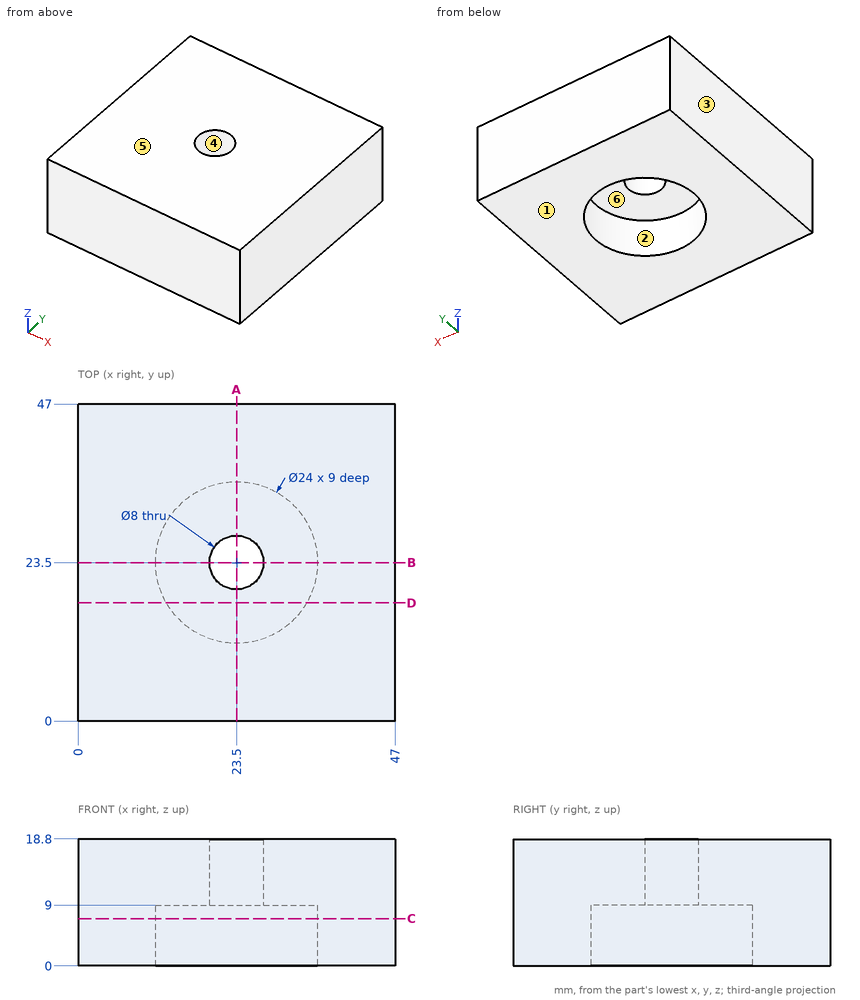
Design review of the part shown in the three views and the two pictorial views. Dimensions are in mm from the part's minimum x, y and z. A direction names the side the tool comes from. Round coordinates to 2 decimals unless told otherwise and drop trailing zeros. Loops run counter-clockwise (first coordinate to the right, second up) from the corner with the lowest first, then second, coordinate; pieces in that order, holes last. Notation, with made-up numbers: (-29, 44) - (7, 44) arc R13 ccw to (7, 65) - close; hole circle Ø5 at (36, 30.5). An arc over 180 degrees is marked (long way). Write each question's results on one line, items separated by ' | '. Start each with the question number.
Q1. Draft analysis for pull direction X (two halves, no side actions). For the marked faces 1, 2, 3 and 4, state which applies: pulls with the +X half, pulls with the -X half, needs draft (parallel to the pull), parting line crosses it, or undercut.
Q2. Take a section at D-D on y = 17.5. Give the boundary of the cut face in (x, z), plus the area to 3 significant figures.
Q3. Tool access review of the marked faces 5 and 6: name each direction out of +Z, -Z, +X, -X, +Y, -Y from which nothing blocks a thin tool from reaching the whole face with its end or side.
Q4. Take a section at A-A on x = 23.5. Give the boundary of the cut face in (y, z).
Q5. Wall thickness on line 1 along Y through (x, z) = (23.5, 2.5); line 2 along Z through (x, y) = (30, 24); line 3 along Y through (x, z) = (12.5, 6): over which ranges is each line inside the solid? List them lowest first. Write a range as [from, to].
Q6. Take a section at C-C on z = 7. Give the boundary of the cut face in (x, y).
Q7. Insertion check: P1, Ø7, axis at x = 17.5, y = 20.5, coming from the -Z side. The pin has a flat end and moves straight along its axis. Give the tip position at first contact, or say it passes through.
Data:
1) face 1: needs draft | face 2: undercut | face 3: pulls with the -X half | face 4: undercut
2) outline: (0, 0) - (13.11, 0) - (13.11, 9) - (33.89, 9) - (33.89, 0) - (47, 0) - (47, 18.8) - (0, 18.8) - close | area: 697 mm²
3) face 5: +Z, +X, -X, +Y, -Y | face 6: -Z
4) outline: (0, 0) - (11.5, 0) - (11.5, 9) - (19.5, 9) - (19.5, 18.8) - (0, 18.8) - close; (27.5, 9) - (35.5, 9) - (35.5, 0) - (47, 0) - (47, 18.8) - (27.5, 18.8) - close
5) line 1: y = [0, 11.5], [35.5, 47] | line 2: z = [9, 18.8] | line 3: y = [0, 18.7], [28.3, 47]
6) outline: (0, 0) - (47, 0) - (47, 47) - (0, 47) - close; hole circle Ø24 at (23.5, 23.5)
7) P1: stops at z = 9
